The model under review builds one solid part; all positions refer to its coordinate system, in mm. Face numbers are marked on the shaded views. Round coordinates to 2 decimals unless told otherwise and drop trailing zeros. Order: outer loops, then holes, each group sorted by start corner. A loop starts at its lowest first (then second) coordinate and runs counter-clockwise, first axis right, second up.
```python
from build123d import *

# Parameters (mm, degrees)
SKETCH1_W           = 350
SKETCH1_H           = 140
BOSS_EXTRUDE1_DEPTH = 140
SKETCH2_R           = 10.5
CUT_EXTRUDE3_DEPTH  = 41
FILLET2_R           = 30
FILLET3_R           = 1
SKETCH3_R           = 10
BOSS_EXTRUDE3_DEPTH = 40


with BuildPart() as part:
    # Sketch1 → Boss-Extrude1 (new body)
    with BuildSketch(Plane(origin=(0, 0, 0), x_dir=(1, 0, 0), z_dir=(0, 1, 0))):
        with Locations((175, -70)):
            Rectangle(SKETCH1_W, SKETCH1_H)
    extrude(amount=BOSS_EXTRUDE1_DEPTH)

    # Sketch2 → Cut-Extrude3 (cut)
    with BuildSketch(Plane(origin=(0, 0, 0), x_dir=(0, 0, -1), z_dir=(1, 0, 0))):
        with Locations((-70, 100)):
            Circle(SKETCH2_R)
        with Locations((-70, 40)):
            Circle(SKETCH2_R)
    extrude(amount=CUT_EXTRUDE3_DEPTH, mode=Mode.SUBTRACT)

    # Fillet2
    fillet2_edges = [part.edges().sort_by_distance(p)[0] for p in [
        (175, 140, 140),
        (175, 0, 140),
    ]]
    fillet(fillet2_edges, radius=FILLET2_R)

    # Fillet3
    fillet3_edges = [part.edges().sort_by_distance(p)[0] for p in [
        (175, 140, 0),
        (175, 0, 0),
    ]]
    fillet(fillet3_edges, radius=FILLET3_R)

    # Sketch3 → Boss-Extrude3 (add)
    with BuildSketch(Plane(origin=(350, 0, 0), x_dir=(0, 0, -1), z_dir=(1, 0, 0))):
        with Locations((-70, 100)):
            Circle(SKETCH3_R)
        with Locations((-70, 40)):
            Circle(SKETCH3_R)
    extrude(amount=BOSS_EXTRUDE3_DEPTH)


solid = part.part
```
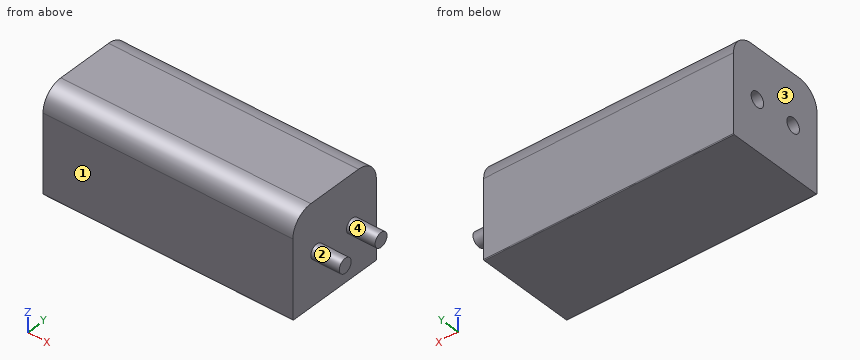
(1) Draft analysis for pull direction Y (two halves, no side actions). For the marked faces 1, 2, 3 and 4, state which applies: pulls with the +Y half, pulls with the -Y half, needs draft (parallel to the pull), parting line crosses it, or undercut.
Data:
face 1: pulls with the -Y half
face 2: undercut
face 3: needs draft
face 4: undercut
(2) Consider section C-C (x = 142). Write out the cut boundary in (y, z), and give its area (3 significant figures).
Data:
outline: (0, 1) arc R1 ccw to (1, 0) - (139, 0) arc R1 ccw to (140, 1) - (140, 110) arc R30 ccw to (110, 140) - (30, 140) arc R30 ccw to (0, 110) - close
area: 19,200 mm2
(3) Consider section D-D (x = 361.5). Write out the cut boundary in (y, z).
Data:
outline: circle Ø20 at (40, 70); circle Ø20 at (100, 70)
(4) Consider section A-A (z = 70). Write out the cut boundary in (x, y).
Data:
outline: (0, 0) - (350, 0) - (350, 30) - (390, 30) - (390, 50) - (350, 50) - (350, 90) - (390, 90) - (390, 110) - (350, 110) - (350, 140) - (0, 140) - (0, 110.5) - (41, 110.5) - (41, 89.5) - (0, 89.5) - (0, 50.5) - (41, 50.5) - (41, 29.5) - (0, 29.5) - close
(5) Insertion check: pin 1 (10.5 mm diameter, centred on y = 96, z = 67, fed in from -X); pin 2 (1.5 mm diameter, centred on y = 119.5, z = 42.5, fed in from +X). Each pin has a flat end and moves straight along its axis. Give the tip position at first contact, or say it passes through.
Data:
pin 1: stops at x = 41
pin 2: stops at x = 350
(6) Consider section B-B (y = 40). Write out the cut boundary in (x, z), and give its area (3 significant figures).
Data:
outline: (0, 0) - (350, 0) - (350, 60) - (390, 60) - (390, 80) - (350, 80) - (350, 140) - (0, 140) - (0, 80.5) - (41, 80.5) - (41, 59.5) - (0, 59.5) - close
area: 48,900 mm2
(7) To check wall thickness, follow probe 1 along Y at (x, z) = (31, 70); probe 2 along X at (y, z) = (8, 64.5); probe 3 along Z at (x, y) = (263.5, 29). State the ranges of each line that lie inside material, in increasing order.
Data:
probe 1: y = 0 to 29.5, 50.5 to 89.5, 110.5 to 140
probe 2: x = 0 to 350
probe 3: z = 0 to 139.98
